Geometry: final body of the model. Coordinates: model frame, mm. Face numbers are marked on the shaded views. A direction names the side the tool comes from. Coordinates: 2 decimals unless noted, no trailing zeros. Loops run counter-clockwise (first coordinate to the right, second up) from the corner with the lowest first, then second, coordinate; pieces in that order, holes last. Notation, with made-up numbers: M -35,0 L 24,0 A24 cw 24,30 Z; hole C 29,-15.75 d7. An arc over 180 degrees is marked long. Write item = value, one per line. Start each with the question number.
```python
from build123d import *

# Parameters (mm, degrees)
SKETCH1_R           = 8.75
SKETCH1_R_2         = 1.5
BOSS_EXTRUDE1_DEPTH = 5
SKETCH1_2_R         = 1.5
BOSS_EXTRUDE2_DEPTH = 10
BOSS_EXTRUDE3_START = 10
SKETCH2_W           = 15
SKETCH2_H           = 27.755893748
SKETCH2_R           = 1.259283935
BOSS_EXTRUDE3_DEPTH = 2
BOSS_EXTRUDE4_START = 6
BOSS_EXTRUDE4_DEPTH = 1
BOSS_EXTRUDE5_START = -6
BOSS_EXTRUDE5_DEPTH = 1


with BuildPart() as part:
    # Sketch1 → Boss-Extrude1 (new, symmetric)
    with BuildSketch(Plane(origin=(0, 0, 0), x_dir=(0, 0, -1), z_dir=(1, 0, 0))):
        Circle(SKETCH1_R)
        Circle(SKETCH1_R_2, mode=Mode.SUBTRACT)
    extrude(amount=BOSS_EXTRUDE1_DEPTH, both=True)

    # Sketch1<2> → Boss-Extrude2 (add, symmetric)
    with BuildSketch(Plane(origin=(0, 0, 0), x_dir=(0, 0, -1), z_dir=(1, 0, 0))):
        Circle(SKETCH1_2_R)
    extrude(amount=BOSS_EXTRUDE2_DEPTH, both=True)



with BuildPart() as body_2:
    # Sketch2 → Boss-Extrude3 (new body)
    with BuildSketch(Plane(origin=(0, 0, 0), x_dir=(1, 0, 0), z_dir=(0, 1, 0)).offset(BOSS_EXTRUDE3_START)):
        Rectangle(SKETCH2_W, SKETCH2_H)
        with Locations((0, 10.696409263)):
            Circle(SKETCH2_R, mode=Mode.SUBTRACT)
        with Locations((0, -10.934061862)):
            Circle(SKETCH2_R, mode=Mode.SUBTRACT)
    extrude(amount=BOSS_EXTRUDE3_DEPTH)


with BuildPart() as part_1:
    add(part.part)

    add(body_2.part)  # Boss-Extrude4 merges body 2
    # Sketch3 → Boss-Extrude4 (add)
    with BuildSketch(Plane(origin=(0, 0, 0), x_dir=(0, 0, -1), z_dir=(1, 0, 0)).offset(BOSS_EXTRUDE4_START)):
        Polygon((-13.877946874, 10), (-2.605119046, -2.991355361), (2.097655879, -2.991355361), (13.877946874, 10), align=None)
    extrude(amount=BOSS_EXTRUDE4_DEPTH)

    # Sketch3<2> → Boss-Extrude5 (add)
    with BuildSketch(Plane(origin=(0, 0, 0), x_dir=(0, 0, -1), z_dir=(1, 0, 0)).offset(BOSS_EXTRUDE5_START)):
        Polygon((-13.877946874, 10), (-2.605119046, -2.991355361), (2.097655879, -2.991355361), (13.877946874, 10), align=None)
    extrude(amount=-BOSS_EXTRUDE5_DEPTH)


solid = part_1.part
```
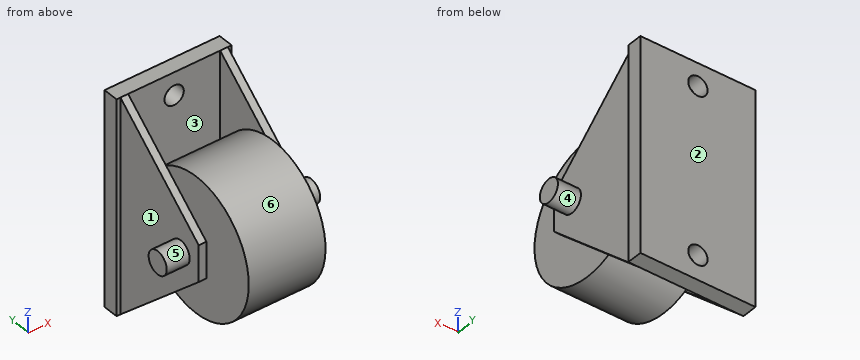
Item 1: Section query D-D (y = 9.25). Return the cut outline in (x, z), plus the area to 4 significant figures.
Item 2: Section query B-B (x = -3.5). Return the cut outline in (y, z).
Item 3: Pull-direction query (Y, two-part tool) for the marked faces 1 and 2; classes: released by +Y, released by -Y, zero draft, split by the parting line, or undercut.
Item 4: Section query A-A (x = 0). Return the cut outline in (y, z).
Item 5: Reachability of the marked faces 3, 4, 5 and 6 from +Z, -Z, +X, -X, +Y, -Y: full face, straight path, thin tool, end or side. Return the list, or none.
Item 6: First-contact query: pin 1 (1.5 mm diameter, centred on x = -0.5, z = 8.5, fed in from -Y); pin 2 (8 mm diameter, centred on x = 0, y = -5.5, fed in from +Z); pin 3 (3.5 mm diameter, centred on x = 2, z = -4.5, fed in from -Y); pin 4 (5 mm diameter, centred on y = -2, z = 0, fed in from +X). Flat tips, straight axial feed; report the tip coordinate or a pass-through.
Item 7: Line query: line 1 (Z direction, x = 0, y = 10.5); line 2 (X direction, y = 3.5, z = 6.5); line 3 (X direction, y = 6.5, z = -9). Output: solid intervals per line, ascending. Write a range as from..to.
Verdict:
q1.outline = M -7,-13.2 L -6,-13.2 L -6,13.23 L -7,13.23 Z; M 6,-13.2 L 7,-13.2 L 7,13.23 L 6,13.23 Z
q1.area = 52.85 mm2
q2.outline = C 0,0 d17.5; M 10,-13.88 L 12,-13.88 L 12,13.88 L 10,13.88 Z
q3.face_1 = undercut
q3.face_2 = released by +Y
q4.outline = C 0,0 d17.5; M 10,-13.88 L 12,-13.88 L 12,-11.96 L 10,-11.96 Z; M 10,-9.44 L 12,-9.44 L 12,9.67 L 10,9.67 Z; M 10,12.19 L 12,12.19 L 12,13.88 L 10,13.88 Z
q5.face_3 = +Z, -Z
q5.face_4 = +X
q5.face_5 = -X
q5.face_6 = none
q6.pin_1 = -4.06
q6.pin_2 = 8.62
q6.pin_3 = -8.31
q6.pin_4 = 10
q7.line_1 = -13.88..-11.96, -9.44..9.67, 12.19..13.88
q7.line_2 = -7..-6, -5..5, 6..7
q7.line_3 = -7..-6, 6..7
